Read the model definition and answer for the solid it produces. Units are mm, in the model's axes. A direction names the side the tool comes from. Coordinates: 2 decimals unless noted, no trailing zeros. Write each loop counter-clockwise with the first axis right and the second up, starting at its lowest first coordinate (ties: lowest second). Pieces come first, ordered by that corner, then holes. Notation, with made-up numbers: (-30.5, -4) -> (13.5, -4) arc R18 ccw to (13.5, 15) -> close; hole circle Ø7 at (64, -3.5). An arc over 180 degrees is marked (long way). One line per item, written item: value. Start each with the question number.
Autodesk Inventor part; units mm, degrees
ref_plane "YZ Plane" through (0, 0, 0) normal (1, 0, 0) x (0, 1, 0)
ref_plane "XZ Plane" through (0, 0, 0) normal (0, 1, 0) x (-1, 0, 0)
ref_plane "XY Plane" through (0, 0, 0) normal (0, 0, 1) x (1, 0, 0)
sketch "Sketch1" plane through (0, 0, 0) normal (0, 0, 1) x (1, 0, 0)
  circle A0 centre (0, 0) radius 1.25
  circle A1 centre (-28.1025, 10.5) radius 1.25
  circle A2 centre (-28.1025, -10.5) radius 1.25
  line L0 (0, 0) -> (-28.1025, 0) construction
  line L1 (-28.1025, 10.5) -> (0, 0) construction
  line L2 (-28.1025, 0) -> (-28.1025, 10.5) construction
  circle A3 centre (0, 0) radius 2.5 construction
  circle A4 centre (-28.1025, 10.5) radius 2.5 construction
  circle A5 centre (-28.1025, -10.5) radius 2.5 construction
  line L3 (0, 0) -> (0, 7) construction
  line L4 (0, 3.5) -> (1, 3.5)
  arc A6 (-26.277, 12.2081) -> (0, 3.5) centre (0, 47.5) ccw
  line L5 (0, -3.5) -> (1, -3.5)
  arc A7 (-20.1367, -3.7476) -> (-20.1367, 3.7476) centre (-22, 0) ccw
  arc A8 (-26.277, 12.2081) -> (-33.7448, 6.3389) centre (-29.2155, 8.2614) ccw
  line L6 (-20.1367, 3.7476) -> (-29.2155, 8.2614)
  arc A9 (-29.2155, 8.2614) -> (-32.7919, 6.449) centre (-30.3285, 6.0228) ccw
  arc A10 (-33.7448, 6.3389) -> (-32.7919, 6.449) centre (-33.2846, 6.5343) ccw
  arc A11 (0, -3.5) -> (-26.277, -12.2081) centre (0, -47.5) ccw
  arc A12 (-33.7448, -6.3389) -> (-26.277, -12.2081) centre (-29.2155, -8.2614) ccw
  line L7 (-20.1367, -3.7476) -> (-29.2155, -8.2614)
  arc A13 (-32.7919, -6.449) -> (-29.2155, -8.2614) centre (-30.3285, -6.0228) ccw
  arc A14 (-32.7919, -6.449) -> (-33.7448, -6.3389) centre (-33.2846, -6.5343) ccw
  line L8 (4, 0.5) -> (4, -0.5)
  arc A15 (4, 0.5) -> (1, 3.5) centre (1, 0.5) ccw
  arc A16 (1, -3.5) -> (4, -0.5) centre (1, -0.5) ccw
  dimension "d0" = 2.5
  dimension "d1" = 10.5
  dimension "d2" = 30
  dimension "d3" = 5
  dimension "d22" = 3.5
  dimension "d32" = 0.5
  dimension "d36" = 22
  dimension "d37" = 2.5
  dimension "d38" = 0.5
  dimension "d47" = 44
  dimension "d48" = 4
  dimension "d49" = 3
extrude "Extrusion1" add sketch "Sketch1" along normal blind 4
properties part number "legFrame_short"
1. A tool of negligible diameter and unlimited length cuts with its end or side. For faces 4 (the face through (3.1, 2.64, 1.97)), 5 (the face through (-24.61, -5.97, 1.97)), from which of +Z, -Z, +X, -X, +Y, -Y can it reach the whole face along a straight path? Write none if from no direction.
2. A cutting plane is placed at D-D on x = -10. Give the vertices of the cut face in (y, z).
3. A cutting plane is placed at B-B on z = 2.5. Give the vertices of the cut face in (x, y), then the cut area to 3 significant figures.
4. A cutting plane is placed at C-C on x = -25. Give the vertices of the cut face in (y, z), then the cut area to 3 significant figures.
5. For a pull along Y with two mould halves and no side action, classify faces 1 (the face through (-15, 0, 4)), 2 (the face through (0.5, -3.5, 2)), 3 (the face through (-24.61, 5.97, 1.97)) as +Y half, -Y half, draft (parallel to the pull), parting line (faces both ways), or undercut.
6. Find the intervals of material crossed by probe 1 along Y at (x, z) = (0, 1.35); probe 2 along Y at (x, z) = (-29, 2.8); probe 3 along Y at (x, z) = (-19, 2.7), in increasing order. Write a range as from..to.
7. A cutting plane is placed at A-A on y = 0. Give the vertices of the cut face in (x, z).
8. Given pin 1 (1.5 mm diameter, centred on x = -12.5, z = 2, fed in from -Y); pin 2 (0.8 mm diameter, centred on x = 0.5, z = 2.5, fed in from -Y), each flat-ended and moving along its own axis, determine where each tip first touches the part or whether it passes through.
Derived:
1. face 4: +Z, -Z, +X, +Y
1. face 5: +Z, -Z
2. outline: (-4.65, 0) -> (4.65, 0) -> (4.65, 4) -> (-4.65, 4) -> close
3. outline: (-33.74, -6.34) arc R4.92 ccw to (-26.28, -12.21) arc R44 cw to (0, -3.5) -> (1, -3.5) arc R3 ccw to (4, -0.5) -> (4, 0.5) arc R3 ccw to (1, 3.5) -> (0, 3.5) arc R44 cw to (-26.28, 12.21) arc R4.92 ccw to (-33.74, 6.34) arc R0.5 ccw to (-32.79, 6.45) arc R2.5 cw to (-29.22, 8.26) -> (-20.14, 3.75) arc R4.19 cw to (-20.14, -3.75) -> (-29.22, -8.26) arc R2.5 cw to (-32.79, -6.45) arc R0.5 ccw to start; hole circle Ø2.5 at (-28.1, -10.5); hole circle Ø2.5 at (-28.1, 10.5); hole circle Ø2.5 at (0, 0)
3. area: 337 mm2
4. outline: (-11.29, 0) -> (-6.17, 0) -> (-6.17, 4) -> (-11.29, 4) -> close; (6.17, 0) -> (11.29, 0) -> (11.29, 4) -> (6.17, 4) -> close
4. area: 41.0 mm2
5. face 1: draft
5. face 2: -Y half
5. face 3: undercut
6. probe 1: y = -3.5..-1.25, 1.25..3.5
6. probe 2: y = -13.18..-11.37, -9.63..-8.15, 8.15..9.63, 11.37..13.18
6. probe 3: y = -7.81..-2.92, 2.92..7.81
7. outline: (-17.81, 0) -> (-1.25, 0) -> (-1.25, 4) -> (-17.81, 4) -> close; (1.25, 0) -> (4, 0) -> (4, 4) -> (1.25, 4) -> close
8. pin 1: stops at y = -5.54
8. pin 2: stops at y = -3.5
